Here's how the part is built. I have some questions about the finished solid (model axes, mm). A direction names the side the tool comes from. Round coordinates to 2 decimals unless told otherwise and drop trailing zeros. Loops run counter-clockwise (first coordinate to the right, second up) from the corner with the lowest first, then second, coordinate; pieces in that order, holes last. Notation, with made-up numbers: M 73.5,28.25 L 82.5,28.25 A29 cw 82.5,67.25 Z; hole C -32,75.25 d10. An arc over 180 degrees is marked long. Answer as a JSON object with one key per item and string values.
from build123d import *

# Parameters (mm, degrees)
F1_DEPTH = 8


with BuildPart() as f1:
    # F0 (on Top) → F1 (new body)
    with BuildSketch(Plane.XY):
        Polygon((4, -36), (4, -24), (12, -16), (20, -24), (20, -36), (24, -36), (24, 0), (20, 0), (12, -8), (4, 0), (0, 0), (0, -36), align=None)
        Polygon((10.343146, -12), (4, -18.343146), (4, -5.656854), align=None, mode=Mode.SUBTRACT)
        Polygon((20, -18.343146), (13.656854, -12), (20, -5.656854), align=None, mode=Mode.SUBTRACT)
    extrude(amount=F1_DEPTH)


solid = f1.part
Item 1: I want a section at C-C, the plane y = -13. Please give me the cut outline in (x, z).
Resolved:
{"outline": "M 0,0 L 4,0 L 4,8 L 0,8 Z; M 9.34,0 L 14.66,0 L 14.66,8 L 9.34,8 Z; M 20,0 L 24,0 L 24,8 L 20,8 Z"}
Item 2: I want a section at D-D, the plane x = 6.75. Please give me the cut outline in (y, z).
Resolved:
{"outline": "M -21.25,0 L -15.59,0 L -15.59,8 L -21.25,8 Z; M -8.41,0 L -2.75,0 L -2.75,8 L -8.41,8 Z"}
Item 3: Please list where these lines run through material, in increasing order: probe 1 along X at (y, z) = (-32, 6.5); probe 2 along X at (y, z) = (-6.5, 2); probe 3 along X at (y, z) = (-6, 6.75). Write a range as from..to.
Resolved:
{"probe 1": "0..4, 20..24", "probe 2": "0..4, 4.84..10.5, 13.5..19.16, 20..24", "probe 3": "0..4, 4.34..10, 14..19.66, 20..24"}
Item 4: I want a section at B-B, the plane z = 2. Please give me the cut outline in (x, y), then the cut area to 3 significant figures.
Resolved:
{"outline": "M 0,-36 L 4,-36 L 4,-24 L 12,-16 L 20,-24 L 20,-36 L 24,-36 L 24,0 L 20,0 L 12,-8 L 4,0 L 0,0 Z; hole M 4,-18.34 L 10.34,-12 L 4,-5.66 Z; hole M 13.66,-12 L 20,-18.34 L 20,-5.66 Z", "area": "464 mm²"}
Item 5: If we mould it in two halves opening along Y, with no side actions, what happens to faces 1 (the face through (16, -4, 4)), 2 (the face through (16, -20, 4)), 3 (the face through (12, -14, 8)), 4 (the face through (20, -12, 4))? For each: pulls with the +Y half, pulls with the -Y half, needs draft (parallel to the pull), parting line crosses it, or undercut.
Resolved:
{"face 1": "pulls with the +Y half", "face 2": "pulls with the -Y half", "face 3": "needs draft", "face 4": "undercut"}
Item 6: On a 3-axis mill with a long thin cutter (end or side, diameter ignored), from which of +Z, -Z, +X, -X, +Y, -Y can I reach the whole of each face in a straight line? I mean faces 5 (the face through (8, -4, 4)), 6 (the face through (2, -36, 4)), 7 (the face through (16.784, -8.873, 3.944)), 8 (the face through (20, -30, 4)). Say none if no direction works.
Resolved:
{"face 5": "+Z, -Z, +Y", "face 6": "+Z, -Z, +X, -X, -Y", "face 7": "+Z, -Z", "face 8": "+Z, -Z, -Y"}
Item 7: I want a section at A-A, the plane y = -5. Please give me the cut outline in (x, z).
Resolved:
{"outline": "M 0,0 L 9,0 L 9,8 L 0,8 Z; M 15,0 L 24,0 L 24,8 L 15,8 Z"}
Item 8: I'm going to push flat-ended pins straight in: pin 1 Ø3 at (x, z) = (17, 3.5) entering from -Y; pin 2 Ø1 at (x, z) = (15, 1.5) entering from +Y. Where does each tip first touch, or does it pass through?
Resolved:
{"pin 1": "y = -22.5", "pin 2": "y = -4.5"}
